Design review of the part built by this model. Coordinates are the model's own, in mm. Face numbers are marked on the shaded views. A direction names the side the tool comes from. Coordinates: 2 decimals unless noted, no trailing zeros. Order: outer loops, then holes, each group sorted by start corner. A loop starts at its lowest first (then second) coordinate and runs counter-clockwise, first axis right, second up. Notation, with made-up numbers: M 65.25,67.5 L 75.25,67.5 A24 cw 75.25,84.5 Z; hole C -32,72.25 d11. An arc over 180 degrees is marked long. Use CSV: the item, a comma, the result in double quotes.
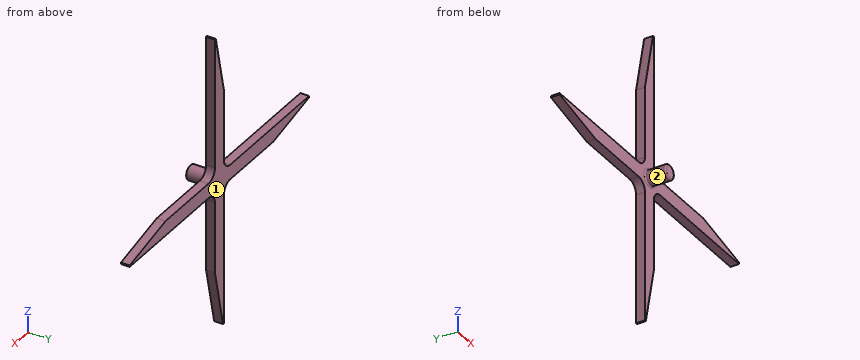
```python
from build123d import *

# Parameters (mm, degrees)
BOSS_EXTRUDE1_DEPTH = 7.62
CUT_EXTRUDE1_DEPTH  = 180.766694357
SKETCH3_R           = 6.35
BOSS_EXTRUDE2_DEPTH = 25.4
FILLET1_R           = 1.27
FILLET2_R           = 1.27


with BuildPart() as part:
    # Sketch1 → Boss-Extrude1 (new body)
    with BuildSketch(Plane(origin=(0, 0, 0), x_dir=(1, 0, 0), z_dir=(0, 1, 0))):
        with BuildLine():
            Line((15.24, 6.35), (127, 6.35))
            Line((127, 6.35), (127, -6.35))
            Line((127, -6.35), (15.24, -6.35))
            ThreePointArc((15.24, -6.35), (8.953820715, -8.953820715), (6.35, -15.24))
            Line((6.35, -15.24), (6.35, -127))
            Line((6.35, -127), (-6.35, -127))
            Line((-6.35, -127), (-6.35, -15.24))
            ThreePointArc((-6.35, -15.24), (-8.953820715, -8.953820715), (-15.24, -6.35))
            Line((-15.24, -6.35), (-127, -6.35))
            Line((-127, -6.35), (-127, 6.35))
            Line((-127, 6.35), (-15.24, 6.35))
            ThreePointArc((-15.24, 6.35), (-8.953820715, 8.953820715), (-6.35, 15.24))
            Line((-6.35, 15.24), (-6.35, 127))
            Line((-6.35, 127), (6.35, 127))
            Line((6.35, 127), (6.35, 15.24))
            ThreePointArc((6.35, 15.24), (8.953820715, 8.953820715), (15.24, 6.35))
        make_face()
    extrude(amount=BOSS_EXTRUDE1_DEPTH)

    # Sketch2 → Cut-Extrude1 (cut, through all)
    with BuildSketch(Plane(origin=(0, 7.62, 0), x_dir=(1, 0, 0), z_dir=(0, 1, 0))):
        Polygon((127, 5.08), (76.2, -6.35), (127, -6.35), align=None)
        Polygon((-5.08, 127), (6.35, 76.2), (6.35, 127), align=None)
        Polygon((5.08, -127), (-6.35, -76.2), (-6.35, -127), align=None)
        Polygon((-127, -5.08), (-76.2, 6.35), (-127, 6.35), align=None)
    extrude(amount=-CUT_EXTRUDE1_DEPTH, mode=Mode.SUBTRACT)

    # Sketch3 → Boss-Extrude2 (add)
    with BuildSketch(Plane(origin=(0, 7.62, 0), x_dir=(1, 0, 0), z_dir=(0, 1, 0))):
        with Locations(Location((0, 0, 0), (0, 0, 270))):
            Circle(SKETCH3_R)
    extrude(amount=-BOSS_EXTRUDE2_DEPTH)

    # Fillet1
    fillet1_edges = [part.edges().sort_by_distance(p)[0] for p in [
        (0, 0, -6.35),
    ]]
    fillet(fillet1_edges, radius=FILLET1_R)

    # Fillet2
    fillet2_edges = [part.edges().sort_by_distance(p)[0] for p in [
        (0, -17.78, -6.35),
    ]]
    fillet(fillet2_edges, radius=FILLET2_R)


solid = part.part
```
(1) Add section D-D on z = -84.5. State the section outline as (x, y) points.
The answers:
outline,"M -6.35,0 L 4.48,0 L 4.48,7.62 L -6.35,7.62 Z"
(2) Add section A-A on z = -19. State the section outline as (x, y) points.
The answers:
outline,"M -6.35,0 L 6.35,0 L 6.35,7.62 L -6.35,7.62 Z"
(3) Add section B-B on y = -7.75. State the section outline as (x, z) points, and give its area (3 significant figures).
The answers:
outline,"C 0,0 d12.7"
area,"127 mm2"
(4) Wall thickness on probe 1 along X at (y, z) = (3.75, 17); probe 2 along Z at (x, y) = (0.5, -4.25): over which ranges is each line inside the solid? List them lowest first.
The answers:
probe 1,"x = -6.35 to 6.35"
probe 2,"z = -6.33 to 6.33"
(5) For the marked faces 1 and 2, list the 3-axis set-ups (+Z, -Z, +X, -X, +Y, -Y) from which the entire face can be reached by the end or side of a thin tool; tool diameter is ignored.
The answers:
face 1,"+Z, -Z, +X, -X, +Y"
face 2,"-Y"
(6) Add section C-C on x = 0. State the section outline as (y, z) points.
The answers:
outline,"M -17.78,-5.08 A1.27 ccw -16.51,-6.35 L -1.27,-6.35 A1.27 cw 0,-7.62 L 0,-104.42 L 7.62,-104.42 L 7.62,104.42 L 0,104.42 L 0,7.62 A1.27 cw -1.27,6.35 L -16.51,6.35 A1.27 ccw -17.78,5.08 Z"
(7) Clearance check with flat-ended pins moving along their axes: P1, Ø4, axis at y = 5, z = 39.5, coming from the -X side; P2, Ø6, axis at x = -91, y = 3, coming from the +Z side; P3, Ø8, axis at y = -7, z = 100, coming from the +X side; P4, Ø2.5, axis at x = -35, y = 4, coming from the -Z side. State where each tip first meets the part, or that it passes through.
The answers:
P1,"stops at x = -6.35"
P2,"stops at z = 6.35"
P3,"passes through"
P4,"stops at z = -6.35"
